```python
from build123d import *

# Parameters (mm, degrees)
F0_R     = 44.5
F0_R_2   = 40
F0_R_3   = 24
F1_DEPTH = 16
F2_DEPTH = 25


with BuildPart() as f1:
    # F0 (on Top) → F1 (new body)
    with BuildSketch(Plane.XY):
        Circle(F0_R)
        Circle(F0_R_2, mode=Mode.SUBTRACT)
        Circle(F0_R_2)
        Circle(F0_R_3, mode=Mode.SUBTRACT)
    extrude(amount=F1_DEPTH)

    # F0 (on Top) → F2 (join)
    with BuildSketch(Plane.XY):
        Circle(F0_R_2)
        Circle(F0_R_3, mode=Mode.SUBTRACT)
    extrude(amount=F2_DEPTH)

    # F3 (on Front) → F4 (revolve, cut)
    with BuildSketch(Plane.XZ):
        Polygon((-34.8, 9.034412), (-44.5, 12), (-44.5, 4), (-34.8, 6.965588), align=None)
    revolve(axis=Axis((0, 0, -5.625665), (0, 0, -1)), mode=Mode.SUBTRACT)


solid = f1.part
```
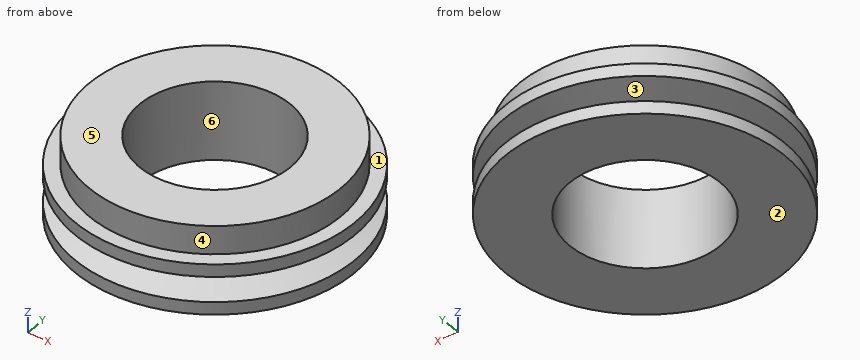
The listing builds one solid part. Answer for the finished solid, in the listing's coordinates (mm). Face numbers are marked on the shaded views. A direction names the side the tool comes from. Coordinates: 2 decimals unless noted, no trailing zeros. Order: outer loops, then holes, each group sorted by start corner. A loop starts at its lowest first (then second) coordinate and runs counter-clockwise, first axis right, second up. Notation, with made-up numbers: M 21.5,35 L 50.5,35 A33 cw 50.5,69 Z; hole C 38,7 d6. An arc over 180 degrees is marked long. Answer as a JSON object with one key per item and string values. Group by question number.
1. A tool of negligible diameter and unlimited length cuts with its end or side. For the marked faces 1, 2 and 3, from which of +Z, -Z, +X, -X, +Y, -Y can it reach the whole face along a straight path? Write none if from no direction.
2. Section C-C on z = 17.5 is taken. Write down the section's boundary in (x, y), then the cut area to 3 significant figures.
3. Flat-ended cylindrical pins translate along their axes: P1, Ø5, axis at x = 8.5, y = 18.5, coming from the +Z side; P2, Ø1, axis at x = -25, z = 21.5, coming from the -Y side; P3, Ø4, axis at y = -14, z = 19, coming from the +X side; P4, Ø10, axis at y = 14.5, z = 21.5, coming from the -X side. Find the tip coordinate at first contact, or state that the pin passes through.
4. Section A-A on y = 0 is taken. Write down the section's boundary in (x, z), then the cut area to 3 significant figures.
5. Determine the mould class of the marked faces 4, 5 and 6 for opening direction Y: released by +Y, released by -Y, zero draft, split by the parting line, or undercut.
6. Straight lines are drawn through the part: line 1 (Y direction, x = 0, z = 16.5); line 2 (Y direction, x = -0.5, z = 13.5); line 3 (X direction, y = -15, z = 15.75) (3 decimals). For each, find the intervals that lie inside material, in ascending order.
Values follow:
{
 "1": {"face 1": "+Z", "face 2": "-Z, +X, -X, +Y, -Y", "face 3": "none"},
 "2": {"outline": "C 0,0 d80; hole C 0,0 d48", "area": "3,220 mm2"},
 "3": {"P1": "through", "P2": "y = -31.62", "P3": "x = 38.16", "P4": "x = -38.86"},
 "4": {"outline": "M -44.5,0 L -24,0 L -24,25 L -40,25 L -40,16 L -44.5,16 L -44.5,12 L -34.8,9.03 L -34.8,6.97 L -44.5,4 Z; M 24,0 L 44.5,0 L 44.5,4 L 34.8,6.97 L 34.8,9.03 L 44.5,12 L 44.5,16 L 40,16 L 40,25 L 24,25 Z", "area": "846 mm2"},
 "5": {"face 4": "split by the parting line", "face 5": "zero draft", "face 6": "undercut"},
 "6": {"line 1": "-40 to -24, 24 to 40", "line 2": "-44.5 to -23.99, 23.99 to 44.5", "line 3": "-41.896 to -18.735, 18.735 to 41.896"}
}
